Input: part model. Units: mm. Frame: model coordinates. A direction names the side the tool comes from. Round coordinates to 2 decimals unless told otherwise and drop trailing zeros. Loops run counter-clockwise (first coordinate to the right, second up) from the corner with the lowest first, then second, coordinate; pieces in that order, holes last. Notation, with made-up numbers: (-26.75, 16) - (-21.75, 16) arc R21 cw to (-21.75, 43) - close; hole circle Ø3 at (-7, 75.25). An arc over 180 degrees is marked (long way). Use CSV: the item, a comma, the result in double quotes. Start each with the question number.
1. Cut plane A-A (y = 50.5). Return loops of the section in (x, z).
2. Access query for faces 5 (the flat face through (-60.5, 34, 0)), 6 (the flat face through (65, 40, -10)), 7 (the flat face through (-75, 35, -8)). Directions: +Z, -Z, +X, -X, +Y, -Y. A direction counts if a zero-diameter tool reaches every point of the face in a straight line with its end or side. Return the directions, or none.
3. Cut plane D-D (x = -70). Return loops of the section in (y, z), and give its area (3 significant figures).
4. Pin query (flat end, axial travel): P1, Ø8, axis at x = -14.5, z = -7.5, coming from the -Y side. Return the tip coordinate at first contact, or that it passes through.
5. Material intervals for probe 1 along X at (y, z) = (24.5, -7.5); probe 2 along Z at (x, y) = (-70, 41); probe 3 along X at (y, z) = (12.5, -12), sorted ascending. Write a range as from..to.
6. Cut plane C-C (z = -7.5). Return loops of the section in (x, y).
7. Pull-direction query (Z, two-part tool) for faces 1 (the cylindrical face through (71.908, 34.983, -8.101)), 2 (the flat face through (5, 7, -16.5)), 3 (the flat face through (-1, 4, 1.5)), 4 (the flat face through (60.5, 34, 0)); classes: +Z half, -Z half, draft (parallel to the pull), parting line (faces both ways), or undercut.
8. Cut plane B-B (x = 31.5). Return loops of the section in (y, z), and give its area (3 significant figures).
```python
from build123d import *

# Parameters (mm, degrees)
SKETCH1_W                = 130
SKETCH1_H                = 3
BOSS_EXTRUDE1_DEPTH      = 69
SKETCH2_W                = 121
SKETCH2_H                = 51
CUT_EXTRUDE1_DEPTH       = 65
BOSS_EXTRUDE3_DEPTH      = 15
BOSS_EXTRUDE3_DEPTH_BACK = 3
SKETCH4_R                = 2
CUT_EXTRUDE2_DEPTH       = 70
FILLET1_R                = 2
FILLET2_R                = 2


with BuildPart() as part:
    # Sketch1 → Boss-Extrude1 (new body)
    with BuildSketch(Plane(origin=(0, 0, 0), x_dir=(1, 0, 0), z_dir=(0, 1, 0))):
        Rectangle(SKETCH1_W, SKETCH1_H)
    extrude(amount=BOSS_EXTRUDE1_DEPTH)

    # Sketch2 → Cut-Extrude1 (cut)
    with BuildSketch(Plane.XY.offset(1.5)):
        with Locations((0, 34.5)):
            Rectangle(SKETCH2_W, SKETCH2_H)
    extrude(amount=-CUT_EXTRUDE1_DEPTH, mode=Mode.SUBTRACT)

    # Sketch3 → Boss-Extrude3 (add, two sides)
    with BuildSketch(Plane(origin=(0, 0, -1.5), x_dir=(-1, 0, 0), z_dir=(0, 0, -1))) as boss_extrude3_sk:
        Polygon((75, 0), (-75, 0), (-75, 69), (-65, 69), (-65, 9), (65, 9), (65, 69), (75, 69), align=None)
    extrude(amount=BOSS_EXTRUDE3_DEPTH)
    extrude(boss_extrude3_sk.sketch, amount=-BOSS_EXTRUDE3_DEPTH_BACK)

    # Sketch4 → Cut-Extrude2 (cut, through all)
    with BuildSketch(Plane(origin=(0, 69, 0), x_dir=(1, 0, 0), z_dir=(0, 1, 0))):
        with Locations((-70, 7.5)):
            Circle(SKETCH4_R)
        with Locations((70, 7.5)):
            Circle(SKETCH4_R)
    extrude(amount=-CUT_EXTRUDE2_DEPTH, mode=Mode.SUBTRACT)

    # Fillet1
    fillet1_edges = [part.edges().sort_by_distance(p)[0] for p in [
        (-65, 9, -9),
        (65, 9, -9),
    ]]
    fillet(fillet1_edges, radius=FILLET1_R)

    # Fillet2
    fillet2_edges = [part.edges().sort_by_distance(p)[0] for p in [
        (-61.75, 9, -1.5),
        (-65, 40, -1.5),
        (61.75, 9, -1.5),
        (65, 40, -1.5),
        (-64.414213562, 9.585786438, -1.5),
        (64.414213562, 9.585786438, -1.5),
    ]]
    fillet(fillet2_edges, radius=FILLET2_R)


solid = part.part
```
Established:
1,outline,"(-75, -16.5) - (-65, -16.5) - (-65, -3.5) arc R2 cw to (-63, -1.5) - (-60.5, -1.5) - (-60.5, 1.5) - (-75, 1.5) - close; (60.5, -1.5) - (63, -1.5) arc R2 cw to (65, -3.5) - (65, -16.5) - (75, -16.5) - (75, 1.5) - (60.5, 1.5) - close; hole circle Ø4 at (-70, -7.5); hole circle Ø4 at (70, -7.5)"
2,face 5,"+Z, -Z"
2,face 6,"-Z, +Y"
2,face 7,"+Z, -Z, -X, +Y, -Y"
3,outline,"(0, -16.5) - (69, -16.5) - (69, -9.5) - (0, -9.5) - close; (0, -5.5) - (69, -5.5) - (69, 1.5) - (0, 1.5) - close"
3,area,"966 mm2"
4,P1,"stops at y = 0"
5,probe 1,"x = -75..-72, -68..-65, 65..68, 72..75"
5,probe 2,"z = -16.5..-9.5, -5.5..1.5"
5,probe 3,"x = -75..-65, 65..75"
6,outline,"(-75, 0) - (-72, 0) - (-72, 69) - (-75, 69) - close; (-68, 0) - (68, 0) - (68, 69) - (65, 69) - (65, 11) arc R2 cw to (63, 9) - (-63, 9) arc R2 cw to (-65, 11) - (-65, 69) - (-68, 69) - close; (72, 0) - (75, 0) - (75, 69) - (72, 69) - close"
7,face 1,"undercut"
7,face 2,"-Z half"
7,face 3,"+Z half"
7,face 4,"draft"
8,outline,"(0, -16.5) - (9, -16.5) - (9, 1.5) - (0, 1.5) - close; (60, -1.5) - (69, -1.5) - (69, 1.5) - (60, 1.5) - close"
8,area,"189 mm2"
